Geometry: final body of the model. Coordinates: model frame, mm. Round coordinates to 2 decimals unless told otherwise and drop trailing zeros. Loops run counter-clockwise (first coordinate to the right, second up) from the corner with the lowest first, then second, coordinate; pieces in that order, holes last. Notation, with made-up numbers: M 73,-28.75 L 119,-28.75 A11 ccw 119,-7.75 Z; hole C -29.5,34.25 d7. An arc over 180 degrees is marked long. Answer as a JSON object with one key per item and string values.
```python
from build123d import *

# Parameters (mm, degrees)
BOSS_EXTRUDE1_DEPTH = 25.4
FILLET1_R           = 12.7
CUT_EXTRUDE1_DEPTH  = 25.4
CUT_EXTRUDE3_DEPTH  = 25.4


with BuildPart() as part:
    # Sketch1 → Boss-Extrude1 (new body)
    with BuildSketch(Plane.XY):
        Polygon((0, 170.18), (5.08, 170.18), (5.08, 5.08), (220.98, 5.08), (220.98, 0), (0, 0), align=None)
    extrude(amount=-BOSS_EXTRUDE1_DEPTH)

    # Fillet1
    fillet1_edges = [part.edges().sort_by_distance(p)[0] for p in [
        (220.98, 2.54, -25.4),
        (220.98, 2.54, 0),
        (2.54, 170.18, -25.4),
        (2.54, 170.18, 0),
    ]]
    fillet(fillet1_edges, radius=FILLET1_R - 0.0001)  # a hair under: the kernel refuses the full size

    # Sketch4 → Cut-Extrude1 (cut)
    with BuildSketch(Plane(origin=(5.08, 0, 0), x_dir=(0, 0, -1), z_dir=(1, 0, 0))):
        with BuildLine():
            Line((9.525, 158.115), (9.525, 18.415))
            ThreePointArc((9.525, 18.415), (12.7, 15.24), (15.875, 18.415))
            Line((15.875, 18.415), (15.875, 158.115))
            ThreePointArc((15.875, 158.115), (12.7, 161.29), (9.525, 158.115))
        make_face()
    extrude(amount=-CUT_EXTRUDE1_DEPTH, mode=Mode.SUBTRACT)

    # Sketch5 → Cut-Extrude3 (cut)
    with BuildSketch(Plane(origin=(0, 5.08, 0), x_dir=(1, 0, 0), z_dir=(0, 1, 0))):
        with BuildLine():
            Line((207.01, 17.78), (16.51, 17.78))
            ThreePointArc((16.51, 17.78), (11.43, 12.7), (16.51, 7.62))
            Line((16.51, 7.62), (207.01, 7.62))
            ThreePointArc((207.01, 7.62), (212.09, 12.7), (207.01, 17.78))
        make_face()
    extrude(amount=-CUT_EXTRUDE3_DEPTH, mode=Mode.SUBTRACT)


solid = part.part
```
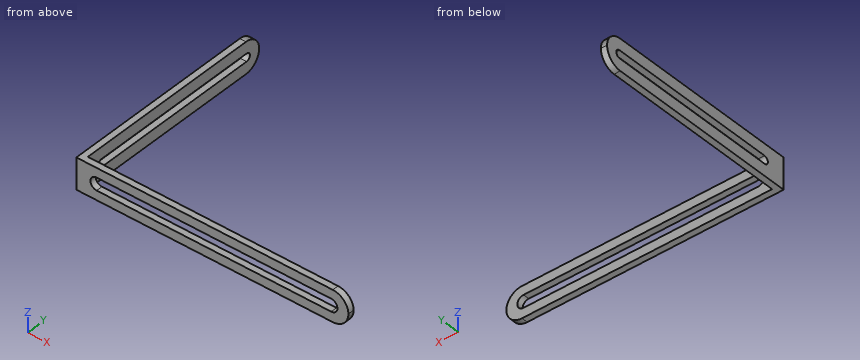
1) Line query: probe 1 along Y at (x, z) = (189, -22). Output: solid intervals per line, ascending.
Geometry results:
{"probe 1": "0 to 5.08"}
2) Cut plane B-B on x = 72. Return the cut outline in (y, z).
Geometry results:
{"outline": "M 0,-25.4 L 5.08,-25.4 L 5.08,-17.78 L 0,-17.78 Z; M 0,-7.62 L 5.08,-7.62 L 5.08,0 L 0,0 Z"}
3) Cut plane C-C on z = -4. Return the cut outline in (x, y), and give its area (3 significant figures).
Geometry results:
{"outline": "M 0,0 L 217.53,0 L 217.53,5.08 L 5.08,5.08 L 5.08,166.73 L 0,166.73 Z", "area": "1,930 mm2"}
4) Cut plane A-A on y = 90. Return the cut outline in (x, z) (3 decimals).
Geometry results:
{"outline": "M 0,-25.4 L 5.08,-25.4 L 5.08,-15.875 L 0,-15.875 Z; M 0,-9.525 L 5.08,-9.525 L 5.08,0 L 0,0 Z"}
5) First-contact query: pin 1 (4 mm diameter, centred on y = 58.5, z = -6, fed in from +X); pin 2 (5 mm diameter, centred on x = 126.5, z = -15, fed in from +Y); pin 3 (3 mm diameter, centred on x = 40.5, z = -4.5, fed in from +Y). Flat tips, straight axial feed; report the tip coordinate or a pass-through.
Geometry results:
{"pin 1": "x = 5.08", "pin 2": "through", "pin 3": "y = 5.08"}
